Design review of the part shown in the three views and the two pictorial views. Dimensions are in mm from the part's minimum x, y and z. A direction names the side the tool comes from. Give positions to 0.01 mm unless a question says otherwise; leave off trailing zeros. Order: outer loops, then holes, each group sorted by start corner. A loop starts at its lowest first (then second) coordinate and runs counter-clockwise, first axis right, second up.
Item 1: For probe 1 along Y at (x, z) = (236, 304); probe 2 along X at (y, z) = (168, 298); probe 3 along Z at (x, y) = (474, 247), list the stretches that pass through material, from the lowest coordinate up.
Item 2: Consider section C-C (z = 138). Give the boundary of the cut face in (x, y), plus the area to 3 significant figures.
Item 3: Consider section B-B (x = 480). Give the boundary of the cut face in (y, z).
Item 4: Consider section A-A (y = 224). Give the boundary of the cut face in (x, z), plus the area to 3 significant figures.
Item 5: Consider section D-D (y = 169). Give the boundary of the cut face in (x, z), plus the area to 3 significant figures.
Item 6: Machinability: for the marked faces 1, 2 and 3, which of the approach directions +Z, -Z, +X, -X, +Y, -Y give a long, thin tool a straight path to every point of the face, cutting with its end or side? Answer none if there is none.
Item 7: For P1, Ø10, axis at y = 137.5, z = 271.5, coming from the -X side; P2, Ø2, axis at y = 119.5, z = 213, coming from the -X side; P3, Ø5, axis at y = 79.5, z = 90.5, coming from the +X side, all flat-tipped, find the tip position at first contact; note any pin that passes through.
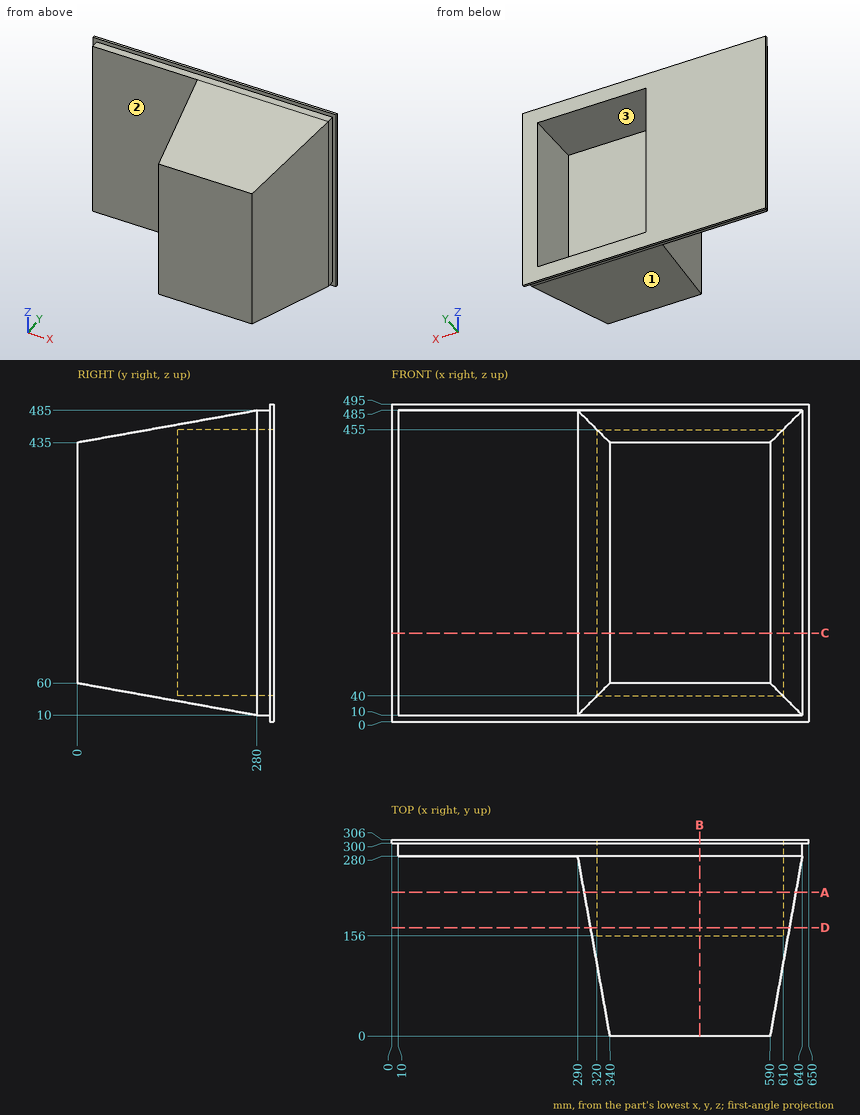
Resolved:
1. probe 1: y = 280 to 306
1. probe 2: x = 310 to 320, 610 to 620
1. probe 3: z = 15.89 to 40, 455 to 479.11
2. outline: (0, 300) - (10, 300) - (10, 280) - (290, 280) - (340, 0) - (590, 0) - (640, 280) - (640, 300) - (650, 300) - (650, 306) - (610, 306) - (610, 156) - (320, 156) - (320, 306) - (0, 306) - close
2. area: 57,000 mm2
3. outline: (0, 60) - (280, 10) - (300, 10) - (300, 0) - (306, 0) - (306, 40) - (156, 40) - (156, 455) - (306, 455) - (306, 495) - (300, 495) - (300, 485) - (280, 485) - (0, 435) - close
4. outline: (300, 20) - (630, 20) - (630, 475) - (300, 475) - close; hole (320, 40) - (610, 40) - (610, 455) - (320, 455) - close
4. area: 29,800 mm2
5. outline: (309.82, 29.82) - (620.18, 29.82) - (620.18, 465.18) - (309.82, 465.18) - close; hole (320, 40) - (610, 40) - (610, 455) - (320, 455) - close
5. area: 14,800 mm2
6. face 1: -Z, +X, -X, -Y
6. face 2: +Z, -Z, -X, -Y
6. face 3: +Y
7. P1: stops at x = 314.55
7. P2: stops at x = 318.48
7. P3: stops at x = 604.64
